CAD build for the part. Positions are in the model's coordinates, mm. Face numbers are marked on the shaded views. A direction names the side the tool comes from. Round coordinates to 2 decimals unless told otherwise and drop trailing zeros. Use a Markdown table: item, result. Add a question column.
(1) Two-plate mould, pull along X, no slides. Class the marked faces 3, 4 and 5: released by +X, released by -X, zero draft, split by the parting line, or undercut.
(2) Wall check: L1, parallel to X at y = 126, z = -62; L2, parallel to Y at x = 33.5, z = -21.5; L3, parallel to X at y = -96.5, z = 60.5. Give the ranges that are in metal, low to high.
(3) Flat gauge pins, fed straight in: P1, Ø12, axis at x = -66, y = 82, coming from the -Z side; P2, Ø4, axis at x = -16.5, y = 84.5, coming from the -Z side; P3, Ø3, axis at x = 67.5, z = -44, coming from the +Y side. Where does each tip first touch, or does it go through?
(4) Which spindle directions (+Z, -Z, +X, -X, +Y, -Y) get a long thin tool onto all of the face, cutting with end or side? Do the marked faces 1 and 2. Say none if no direction does.
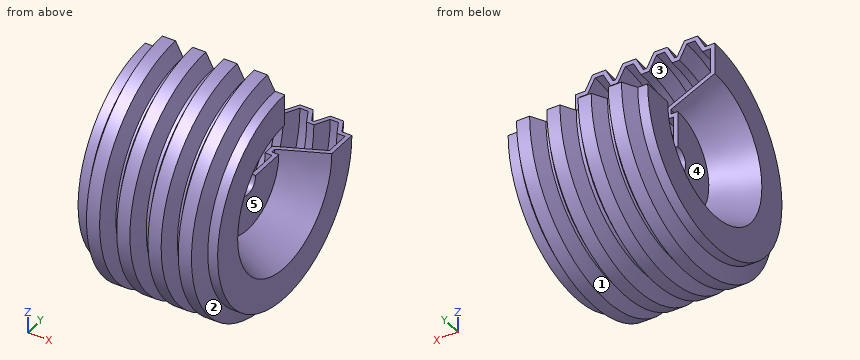
from build123d import *

# Parameters (mm, degrees)
REVOLVE_THIN1_ANGLE = 270


with BuildPart() as part:
    # Sketch1 → Revolve-Thin1 (revolve)
    with BuildSketch(Plane.XY):
        Polygon((-1.995696905, 127.895205728), (-11.034757243, 144.895205728), (-27.043363433, 144.895205728), (-36.082423772, 127.895205728), (-38.917576228, 127.895205728), (-47.956636567, 144.895205728), (-63.965242757, 144.895205728), (-73.004303095, 127.895205728), (-85, 127.895205728), (-85, 89.709854424), (-31.5, 64.762394712), (-31.5, 59), (-40, 59), (-40, 15), (40, 15), (40, 59), (31.5, 59), (31.5, 64.762394712), (85, 89.709854424), (85, 127.895205728), (73.004303095, 127.895205728), (63.965242757, 144.895205728), (47.956636567, 144.895205728), (38.917576228, 127.895205728), (36.082423772, 127.895205728), (27.043363433, 144.895205728), (11.034757243, 144.895205728), (1.995696905, 127.895205728), align=None)
        Polygon((-5, 122.895205728), (-14.039060338, 139.895205728), (-24.039060338, 139.895205728), (-33.078120676, 122.895205728), (-41.921879324, 122.895205728), (-50.960939662, 139.895205728), (-60.960939662, 139.895205728), (-70, 122.895205728), (-80, 122.895205728), (-80, 92.895205728), (-26.5, 67.947746016), (-26.5, 54), (-35, 54), (-35, 20), (35, 20), (35, 54), (26.5, 54), (26.5, 67.947746016), (80, 92.895205728), (80, 122.895205728), (70, 122.895205728), (60.960939662, 139.895205728), (50.960939662, 139.895205728), (41.921879324, 122.895205728), (33.078120676, 122.895205728), (24.039060338, 139.895205728), (14.039060338, 139.895205728), (5, 122.895205728), align=None, mode=Mode.SUBTRACT)
    revolve(axis=Axis((0, 0, 0), (-1, 0, 0)), revolution_arc=REVOLVE_THIN1_ANGLE)


solid = part.part
Return value:
| question | item | result |
|---|---|---|
| 1 | face 3 | undercut |
| 1 | face 4 | released by -X |
| 1 | face 5 | released by +X |
| 2 | L1 | -66.34 to -45.58, -29.42 to -8.66, 8.66 to 29.42, 45.58 to 66.34 |
| 2 | L2 | -131 to -121, -67.89 to -62.08, -54.94 to -49.54, 49.54 to 54.94, 62.08 to 67.89, 121 to 131 |
| 2 | L3 | -85 to -80, 80 to 85 |
| 3 | P1 | z = -123.14 |
| 3 | P2 | z = -119.11 |
| 3 | P3 | y = 134.07 |
| 4 | face 1 | none |
| 4 | face 2 | +X |
